Verification items for the finished model (mm, model axes). Round coordinates to 2 decimals unless told otherwise and drop trailing zeros. Write each loop counter-clockwise with the first axis right and the second up, starting at its lowest first coordinate (ties: lowest second). Pieces come first, ordered by that corner, then holes. Notation, with made-up numbers: (37, -12.75) - (42, -12.75) arc R24 cw to (42, 6.25) - close; hole circle Ø11 at (-36.75, 64). An arc over 180 degrees is marked (long way). Answer as a JSON object with one key per item and string values.
```python
from build123d import *

# Parameters (mm, degrees)
SKETCH1_W           = 6.8
SKETCH1_H           = 7.7
BOSS_EXTRUDE1_DEPTH = 3.95
CUT_EXTRUDE4_START  = -0.275354201
CUT_EXTRUDE4_DEPTH  = 0.275354201


# Read off the part's stored shape, not the designer's step: Cut-Extrude4
with BuildPart() as part:
    # Sketch1 → Boss-Extrude1 (new body)
    with BuildSketch(Plane(origin=(0, 0, 0), x_dir=(1, 0, 0), z_dir=(0, 1, 0))):
        with Locations((3.4, 3.85)):
            Rectangle(SKETCH1_W, SKETCH1_H)
    extrude(amount=BOSS_EXTRUDE1_DEPTH)

    # Cut-Extrude4 outline → Cut-Extrude4 (cut)
    with BuildSketch(Plane(origin=(6.8, 0, 0), x_dir=(0, 0, -1), z_dir=(1, 0, 0)).offset(CUT_EXTRUDE4_START)):
        with BuildLine():
            Line((4.98352639, 3.235480271), (2.901682517, 3.235480271))
            ThreePointArc((2.901682517, 3.235480271), (1.50879417, 1.842591924), (2.901682517, 0.449703578))
            Line((2.901682517, 0.449703578), (4.98352639, 0.449703578))
            ThreePointArc((4.98352639, 0.449703578), (6.376414736, 1.842591924), (4.98352639, 3.235480271))
        make_face()
    extrude(amount=CUT_EXTRUDE4_DEPTH, mode=Mode.SUBTRACT)


solid = part.part
```
1. Material ranges on probe 1 along X at (y, z) = (2, -2.25), recorded low to high. Write a range as from..to.
Completed:
{"probe 1": "x = 0..6.52"}
2. Cross-section at B-B (y = 2.7). Record the boundary of the cut face in (x, z), plus the area to 3 significant figures.
Completed:
{"outline": "(0, -7.7) - (6.8, -7.7) - (6.8, -6.08) - (6.52, -6.08) - (6.52, -1.8) - (6.8, -1.8) - (6.8, 0) - (0, 0) - close", "area": "51.2 mm^2"}
3. Go/stop test with a flat-tipped pin: pin 1 (2 mm diameter, centred on y = 1.5, z = -4.5, fed in from +X). Record where the tip stops, or that it passes through.
Completed:
{"pin 1": "stops at x = 6.52"}
4. Mould release check, pull along Y, two halves, no side actions. Record for faces 1 (the face through (6.525, 2, -4)), 2 (the face through (0, 2, -4)), 3 (the face through (3, 3.95, -4)): released by +Y, released by -Y, zero draft, split by the parting line, or undercut.
Completed:
{"face 1": "undercut", "face 2": "zero draft", "face 3": "released by +Y"}
5. Cross-section at A-A (z = -4). Record the boundary of the cut face in (x, y).
Completed:
{"outline": "(0, 0) - (6.8, 0) - (6.8, 0.45) - (6.52, 0.45) - (6.52, 3.24) - (6.8, 3.24) - (6.8, 3.95) - (0, 3.95) - close"}
